Source: CAD feature listing. Evaluate the final solid. Frame: model axes, mm. Face numbers are marked on the shaded views. A direction names the side the tool comes from. Give positions to 0.01 mm unless a question says otherwise; leave off trailing zeros. Loops run counter-clockwise (first coordinate to the right, second up) from the corner with the lowest first, then second, coordinate; pieces in that order, holes last. Notation, with made-up numbers: (4, 75) -> (59, 75) arc R6 ccw to (59, 85) -> close; hole circle Ø2 at (-26, 39.25). An arc over 180 degrees is marked (long way). Return JSON: item names as keys, results as strings. Group by question number.
(1) Cut plane B-B on z = 55. Return loops of the section in (x, y), then the cut area to 3 significant figures.
(2) Pin query (flat end, axial travel): pin 1 (12 mm diameter, centred on x = -39.5, y = 51, fed in from -Z); pin 2 (3 mm diameter, centred on x = -32.5, y = 85, fed in from +Z); pin 3 (15 mm diameter, centred on x = 55, z = 55, fed in from +Y). Return the tip coordinate at first contact, or that it passes through.
(3) Ray query, line 1 (X direction, y = 2, z = -55); line 2 (X direction, y = 41.5, z = 17); line 3 (Z direction, x = -24.5, y = 59.5). Return the intervals inside material, ascending. Write a range as from..to.
(4) Cut plane C-C on z = 0. Return loops of the section in (x, y), then the cut area to 3 significant figures.
(5) Draft query along X for the marked faces 4, 5 and 6. Return one class per face: released by +X, released by -X, zero draft, split by the parting line, or undercut.
(6) Cut plane D-D on x = 6. Return loops of the section in (y, z).
(7) Cut plane A-A on x = 55. Return loops of the section in (y, z), then the cut area to 3 significant figures.
(8) Access query for the marked faces 1, 2 and 3. Directions: +Z, -Z, +X, -X, +Y, -Y. A direction counts if a zero-diameter tool reaches every point of the face in a straight line with its end or side. Return the directions, or none.
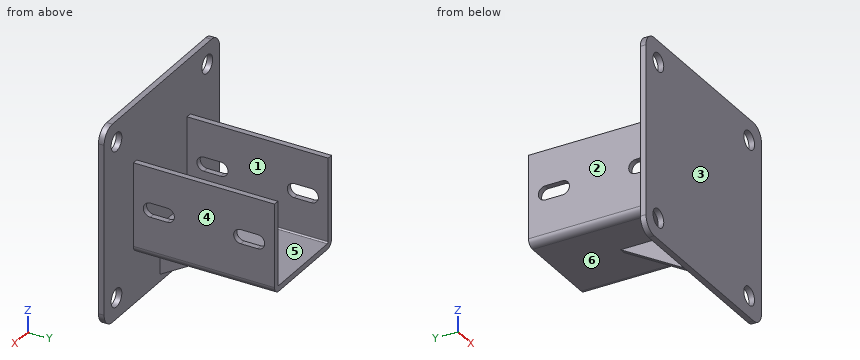
```python
from build123d import *

# Parameters (mm, degrees)
SKETCH_2_W          = 140
SKETCH_2_H          = 140
EXTRUDE_1_DEPTH     = 4
EXTRUDE_1_2_DEPTH   = 100
EXTRUDE_2_DEPTH     = 2
CUT_EXTRUDE_1_DEPTH = 105.5
SKETCH_6_R          = 6.5
CUT_EXTRUDE_2_DEPTH = 5
FILLET_1_R          = 10


with BuildPart() as part:
    # Эскиз2 → Extrude 1 (new body)
    with BuildSketch(Plane(origin=(0, 0, 0), x_dir=(1, 0, 0), z_dir=(0, 1, 0))):
        Rectangle(SKETCH_2_W, SKETCH_2_H)
    extrude(amount=EXTRUDE_1_DEPTH)

    # Эскиз3 → Extrude 1 2 (add)
    with BuildSketch(Plane(origin=(0, 4, 0), x_dir=(1, 0, 0), z_dir=(0, 1, 0))):
        with BuildLine():
            Line((-30.5, -30), (-30.5, 29))
            ThreePointArc((-30.5, 29), (-30.207106781, 29.707106781), (-29.5, 30))
            Line((-29.5, 30), (29.5, 30))
            ThreePointArc((29.5, 30), (30.207106781, 29.707106781), (30.5, 29))
            Line((30.5, 29), (30.5, -30))
            Line((30.5, -30), (34.5, -30))
            Line((34.5, -30), (34.5, 29))
            ThreePointArc((34.5, 29), (33.035533906, 32.535533906), (29.5, 34))
            Line((29.5, 34), (-29.5, 34))
            ThreePointArc((-29.5, 34), (-33.035533906, 32.535533906), (-34.5, 29))
            Line((-34.5, 29), (-34.5, -30))
            Line((-34.5, -30), (-30.5, -30))
        make_face()
    extrude(amount=EXTRUDE_1_2_DEPTH)

    # Эскиз4 → Бобышка-Вытянуть2 (add, symmetric)
    with BuildSketch(Plane(origin=(0, 0, 0), x_dir=(0, 0, -1), z_dir=(1, 0, 0))):
        Polygon((34, 57.693575035), (65, 4), (34, 4), align=None)
    extrude(amount=EXTRUDE_2_DEPTH, both=True)

    # Эскиз5 → Вырез-Вытянуть1 (cut, through all)
    with BuildSketch(Plane(origin=(34.5, 0, 0), x_dir=(0, 0, -1), z_dir=(1, 0, 0))):
        with BuildLine():
            Line((5, 92), (5, 80))
            ThreePointArc((5, 80), (0, 75), (-5, 80))
            Line((-5, 80), (-5, 92))
            ThreePointArc((-5, 92), (0, 97), (5, 92))
        make_face()
        with BuildLine():
            Line((5, 28), (5, 16))
            ThreePointArc((5, 16), (0, 11), (-5, 16))
            Line((-5, 16), (-5, 28))
            ThreePointArc((-5, 28), (0, 33), (5, 28))
        make_face()
    extrude(amount=-CUT_EXTRUDE_1_DEPTH, mode=Mode.SUBTRACT)

    # Эскиз6 → Вырез-Вытянуть2 (cut, through all)
    with BuildSketch(Plane(origin=(0, 4, 0), x_dir=(1, 0, 0), z_dir=(0, 1, 0))):
        with Locations(Location((-55, 55, 0), (0, 0, 270))):  # turned: the seam where the file's is
            Circle(SKETCH_6_R)
        with Locations(Location((-55, -55, 0), (0, 0, 270))):  # turned: the seam where the file's is
            Circle(SKETCH_6_R)
        with Locations(Location((55, 55, 0), (0, 0, 270))):  # turned: the seam where the file's is
            Circle(SKETCH_6_R)
        with Locations(Location((55, -55, 0), (0, 0, 270))):  # turned: the seam where the file's is
            Circle(SKETCH_6_R)
    extrude(amount=-CUT_EXTRUDE_2_DEPTH, mode=Mode.SUBTRACT)

    # Скругление1
    fillet_1_edges = [part.edges().sort_by_distance(p)[0] for p in [
        (70, 2, 70),
        (-70, 2, 70),
        (-70, 2, -70),
        (70, 2, -70),
    ]]
    fillet(fillet_1_edges, radius=FILLET_1_R)


solid = part.part
```
Answers:
{
 "1": {"outline": "(-70, 0) -> (-61.5, 0) -> (-61.5, 4) -> (-70, 4) -> close; (-48.5, 0) -> (48.5, 0) -> (48.5, 4) -> (-48.5, 4) -> close; (61.5, 0) -> (70, 0) -> (70, 4) -> (61.5, 4) -> close", "area": "456 mm²"},
 "2": {"pin 1": "z = -32", "pin 2": "z = 30", "pin 3": "y = 4"},
 "3": {"line 1": "-70..-61.5, -48.5..48.5, 61.5..70", "line 2": "-34.5..-30.5, 30.5..34.5", "line 3": "-34..-30"},
 "4": {"outline": "(-70, 0) -> (70, 0) -> (70, 4) -> (34.5, 4) -> (34.5, 11) -> (30.5, 11) -> (30.5, 4) -> (-30.5, 4) -> (-30.5, 11) -> (-34.5, 11) -> (-34.5, 4) -> (-70, 4) -> close; (-34.5, 33) -> (-30.5, 33) -> (-30.5, 75) -> (-34.5, 75) -> close; (-34.5, 97) -> (-30.5, 97) -> (-30.5, 104) -> (-34.5, 104) -> close; (30.5, 33) -> (34.5, 33) -> (34.5, 75) -> (30.5, 75) -> close; (30.5, 97) -> (34.5, 97) -> (34.5, 104) -> (30.5, 104) -> close", "area": "1,010 mm²"},
 "5": {"face 4": "released by +X", "face 5": "undercut", "face 6": "zero draft"},
 "6": {"outline": "(0, -70) -> (4, -70) -> (4, -34) -> (104, -34) -> (104, -30) -> (4, -30) -> (4, 70) -> (0, 70) -> close"},
 "7": {"outline": "(0, -70) -> (4, -70) -> (4, -61.5) -> (0, -61.5) -> close; (0, -48.5) -> (4, -48.5) -> (4, 48.5) -> (0, 48.5) -> close; (0, 61.5) -> (4, 61.5) -> (4, 70) -> (0, 70) -> close", "area": "456 mm²"},
 "8": {"face 1": "+Z, +Y", "face 2": "+Z, -Z, -X, +Y", "face 3": "+Z, -Z, +X, -X, -Y"}
}
